Could you check a few things on this model? Use its own coordinates, in mm. A direction names the side the tool comes from. Give positions to 0.01 mm unless a question says otherwise; leave off trailing zeros.
(1) On a 3-axis mill with a long thin cutter (end or side, diameter ignored), from which of +Z, -Z, +X, -X, +Y, -Y can I reach the whole of each face in a straight line? I mean faces 1 (the flat face through (-17, 31, 9)), 2 (the cylindrical face through (-12.09, 69.92, 1.75)), 3 (the flat face through (11, 76.832, 3)). Say none if no direction works.
(2) Will these pins go through, and if not, where does the flat tip stop? pin 1 (1.3 mm diameter, centred on x = -17.5, z = 2.5, fed in from +Y); pin 2 (6 mm diameter, centred on x = -11.31, y = 73.43, fed in from +Z); pin 3 (1 mm diameter, centred on y = 13, z = 1.5, fed in from +X); pin 4 (2 mm diameter, centred on x = -12, y = -10, fed in from +Z).
(3) If we mould it in two halves opening along Y, with no side actions, what happens to faces 4 (the cylindrical face through (70.41, 69.92, 1.75)), 5 (the cylindrical face through (75.191, -13.142, 1.014)), 6 (the flat face through (30, -14, 5))? For each: released by +Y, released by -Y, zero draft, split by the parting line, or undercut.
(4) Imagine slicing it at A-A, the plane y = 72. State how many separate pieces and enclosed holes the cut face has, then the cut area to 3 significant figures.
(5) If I drill on probe 1 along Y at (x, z) = (2, 4.75); probe 2 along X at (y, z) = (45, 7); probe 3 along Y at (x, z) = (29.5, 1.75), over which ranges is the centre line in solid material (lowest first)?
from build123d import *

# Parameters (mm, degrees)
F0_W       = 93.5
F0_H       = 93.5
F0_R       = 2.55
F0_R_2     = 43.5
F1_DEPTH   = 2
F3_START   = -10
F3_DEPTH   = 72.5
F4_SIZE    = 1
F6_DEPTH   = 3
F7_SIZE    = 2.99999
F8_R       = 3.6
F9_DEPTH   = 0.5
F10_SIZE   = 1
F11_R      = 5
F12_SIZE   = 1
F13_SIZE   = 0.3
F14_DEPTH  = 0.4
F15_DEPTH  = 0.4
F15_FACE_W = 0.4
F15_FACE_H = 72.5
F14_FACE_W = 0.4
F14_FACE_H = 72.5


# Not quite as in the source:
# - a fillet or chamfer is up to 0.001 mm smaller than in the source, because OpenCascade refuses the exact size


with BuildPart() as f1:
    # F0 (on Top) → F1 (new body)
    with BuildSketch(Plane.XY):
        with Locations((29.9444539048, 32.1819351325)):
            Rectangle(F0_W, F0_H)
        with Locations((-11.3055460952, -9.0680648675)):
            Circle(F0_R, mode=Mode.SUBTRACT)
        with Locations((71.1944539048, -9.0680648675)):
            Circle(F0_R, mode=Mode.SUBTRACT)
        with Locations((29.9444539048, 32.1819351325)):
            Circle(F0_R_2, mode=Mode.SUBTRACT)
        with Locations((-11.3055460952, 73.4319351325)):
            Circle(F0_R, mode=Mode.SUBTRACT)
        with Locations((71.1944539048, 73.4319351325)):
            Circle(F0_R, mode=Mode.SUBTRACT)
    extrude(amount=F1_DEPTH)

    # F2 (on face) → F3 (join)
    with BuildSketch(Plane.XZ.offset(14.5680648675).offset(F3_START)):
        Polygon((-16.8055460952, 9), (-16.2269746666, 6.3), (-14.3147795447, 6.7097560976), (-14.8055460952, 9), align=None)
        Polygon((-16.8055460952, 2), (-15.3055460952, 2), (-16.2269746666, 6.3), (-16.8055460952, 9), (-18.3055460952, 9), align=None)
        Polygon((76.1158824762, 6.3), (75.1944539048, 2), (76.6944539048, 2), (78.1944539048, 9), (76.6944539048, 9), align=None)
        Polygon((74.2036873543, 6.7097560976), (76.1158824762, 6.3), (76.6944539048, 9), (74.6944539048, 9), align=None)
    extrude(amount=-F3_DEPTH)

    # F4
    f4_edges = [f1.edges().sort_by_distance(p)[0] for p in [
        (-14.805546, 31.681935, 9),
        (74.694454, 31.681935, 9),
    ]]
    chamfer(f4_edges, length=F4_SIZE)

    # F5 (on face) → F6 (join)
    with BuildSketch(Plane.XY.offset(2)):
        Polygon((-6.0960170065, -14.5680648675), (66.6944539048, -14.5680648675), (66.6944539048, -12.4680648675), (31.5492184492, -12.4680648675), (31.5492184492, -13.4680648675), (29.0492184492, -13.4680648675), (29.0492184492, -12.4680648675), (-6.0960170065, -12.4680648675), align=None)
        Polygon((66.6944539048, 76.8319351325), (66.6944539048, 78.9319351325), (-6.8055460952, 78.9319351325), (-6.8055460952, 76.8319351325), (28.6944539048, 76.8319351325), (28.6944539048, 77.8319351325), (31.1944539048, 77.8319351325), (31.1944539048, 76.8319351325), align=None)
    extrude(amount=F6_DEPTH)

    # F7 (size 3 in the source; OpenCascade refuses exactly that, so slightly less here)
    f7_edges = [f1.edges().sort_by_distance(p)[0] for p in [
        (66.694454, -13.518065, 5),
        (-6.096017, -13.518065, 5),
        (-6.805546, 77.881935, 5),
        (66.694454, 77.881935, 5),
    ]]
    chamfer(f7_edges, length=F7_SIZE)

    # F8 (on face) → F9 (cut)
    with BuildSketch(Plane.XY.offset(2)):
        with Locations((-11.3055460952, -9.0680648675)):
            Circle(F8_R)
        with Locations((71.1944539048, -9.0680648675)):
            Circle(F8_R)
        with Locations((71.1944539048, 73.4319351325)):
            Circle(F8_R)
        with Locations((-11.3055460952, 73.4319351325)):
            Circle(F8_R)
    extrude(amount=-F9_DEPTH, mode=Mode.SUBTRACT)

    # F10
    f10_edges = [f1.edges().sort_by_distance(p)[0] for p in [
        (-13.855546, -9.068065, 1.5),
        (68.644454, -9.068065, 1.5),
        (68.644454, 73.431935, 1.5),
        (-13.855546, 73.431935, 1.5),
    ]]
    chamfer(f10_edges, length=F10_SIZE)

    # F11
    f11_edges = [f1.edges().sort_by_distance(p)[0] for p in [
        (-16.805546, 78.931935, 1),
        (-16.805546, -14.568065, 1),
        (76.694454, -14.568065, 1),
        (76.694454, 78.931935, 1),
    ]]
    fillet(f11_edges, radius=F11_R)

    # F12
    f12_edges = [f1.edges().sort_by_distance(p)[0] for p in [
        (-13.555546, 32.181935, 0),
    ]]
    chamfer(f12_edges, length=F12_SIZE)

    # F13
    f13_edges = [f1.edges().sort_by_distance(p)[0] for p in [
        (-14.31478, 31.681935, 6.709756),
        (74.203687, 31.681935, 6.709756),
    ]]
    chamfer(f13_edges, length=F13_SIZE)

    # F14 (add): a face of the model
    f14_faces = [f1.faces().sort_by_distance(p)[0] for p in [
        (-17.5555460952, 31.6819351325, 5.5),
    ]]
    extrude(f14_faces, amount=F14_DEPTH)

    # F15 (add): a face of the model
    f15_faces = [f1.faces().sort_by_distance(p)[0] for p in [
        (77.4444539048, 31.6819351325, 5.5),
    ]]
    extrude(f15_faces, amount=F15_DEPTH)

    # F15_face (on face) → F16 (join, up to the next surface of F1)
    with BuildSketch(Plane(origin=(76.8900143876, 31.6819351325, 1.9580941823), x_dir=(1, 0, 0), z_dir=(-0.2095290887, 0, -0.9778024141))):
        Rectangle(F15_FACE_W, F15_FACE_H)
    extrude(until=Until.NEXT)

    # F14_face (on face) → F17 (join, up to the next surface of F1)
    with BuildSketch(Plane(origin=(-17.001106578, 31.6819351325, 1.9580941823), x_dir=(1, 0, 0), z_dir=(0.2095290887, 0, -0.9778024141))):
        Rectangle(F14_FACE_W, F14_FACE_H)
    extrude(until=Until.NEXT)


solid = f1.part
Answer block:
1. face 1: +Z, +X, -X, +Y, -Y
1. face 2: +Z
1. face 3: +Z, +X, -X
2. pin 1: stops at y = 67.93
2. pin 2: stops at z = 0.95
2. pin 3: stops at x = 77.1
2. pin 4: passes through
3. face 4: undercut
3. face 5: released by -Y
3. face 6: zero draft
4. separate pieces: 4
4. enclosed holes: 0
4. area: 93.0 mm2
5. probe 1: y = -14.57 to -12.47, 76.83 to 78.93
5. probe 2: x = -18.29 to -14.38, 74.27 to 78.17
5. probe 3: y = -14.57 to -11.32, 75.68 to 78.93
